from build123d import *

# Parameters (mm, degrees)
CROQUIS1_R              = 1.5875
SALIENTE_EXTRUIR1_DEPTH = 3.175
CORTAR_EXTRUIR1_DEPTH   = 3.175
CORTAR_EXTRUIR3_DEPTH   = 10
CORTAR_EXTRUIR4_DEPTH   = 10
BOSS_EXTRU_1_DEPTH      = 8.18
CONG_1_R                = 2
CONG_2_R                = 3


with BuildPart() as part:
    # Croquis1 → Saliente-Extruir1 (new body)
    with BuildSketch(Plane(origin=(0, 0, 0), x_dir=(1, 0, 0), z_dir=(0, 1, 0))):
        with BuildLine():
            Line((-12.5, 0), (-12.5, -40))
            Line((-12.5, -40), (-2.975, -40))
            Line((-2.975, -40), (-2.975, -20))
            ThreePointArc((-2.975, -20), (-0.046067812, -12.928932188), (7.025, -10))
            Line((7.025, -10), (12.5, -10))
            Line((12.5, -10), (12.5, 40))
            Line((12.5, 40), (2.5, 40))
            Line((2.5, 40), (-12.5, 0))
        make_face()
        with Locations(Location((-7.7375, -5, 0), (0, 0, 270))):
            Circle(CROQUIS1_R, mode=Mode.SUBTRACT)
        with Locations(Location((-7.7375, -35, 0), (0, 0, 270))):
            Circle(CROQUIS1_R, mode=Mode.SUBTRACT)
    extrude(amount=SALIENTE_EXTRUIR1_DEPTH)

    # Croquis2 → Cortar-Extruir1 (cut)
    with BuildSketch(Plane(origin=(0, 3.175, 0), x_dir=(1, 0, 0), z_dir=(0, 1, 0))):
        Polygon((12.5, -10), (6.1, 40), (12.5, 40), align=None)
    extrude(amount=-CORTAR_EXTRUIR1_DEPTH, mode=Mode.SUBTRACT)

    # Croquis3 → Cortar-Extruir3 (cut)
    with BuildSketch(Plane(origin=(0, 3.175, 0), x_dir=(1, 0, 0), z_dir=(0, 1, 0))):
        with BuildLine():
            ThreePointArc((-5.975, -30.575635639), (-7.7375, -30.2375), (-9.5, -30.575635639))
            Line((-9.5, -30.575635639), (-9.5, -9.427055314))
            ThreePointArc((-9.5, -9.427055314), (-7.7375, -9.765), (-5.975, -9.427055314))
            Line((-5.975, -9.427055314), (-5.975, -14.803847577))
            Line((-5.975, -14.803847577), (-5.975, -30.575635639))
        make_face()
        with BuildLine():
            ThreePointArc((-12.5, -35), (-7.7375, -39.7625), (-2.975, -35))
            Line((-2.975, -35), (-2.975, -40))
            Line((-2.975, -40), (-12.5, -40))
            Line((-12.5, -40), (-12.5, -35))
        make_face()
    extrude(amount=-CORTAR_EXTRUIR3_DEPTH, mode=Mode.SUBTRACT)

    # Croquis4 → Cortar-Extruir4 (cut)
    with BuildSketch(Plane(origin=(0, 3.175, 0), x_dir=(1, 0, 0), z_dir=(0, 1, 0))):
        Polygon((7.025, -10), (11.878723404, -5.146276596), (12.5, -10), align=None)
    extrude(amount=-CORTAR_EXTRUIR4_DEPTH, mode=Mode.SUBTRACT)

    # Esquisse1 → Boss.-Extru.1 (add)
    with BuildSketch(Plane(origin=(0, 3.175, 0), x_dir=(1, 0, 0), z_dir=(0, 1, 0))):
        Polygon((11.878723404, -5.146276596), (6.1, 40), (2.5, 40), (8.687234043, -8.337765957), align=None)
    extrude(amount=-BOSS_EXTRU_1_DEPTH)

    # Congé1
    cong_1_edges = [part.edges().sort_by_distance(p)[0] for p in [
        (5.593617021, -5.005, -15.831117021),
    ]]
    fillet(cong_1_edges, radius=CONG_1_R)

    # Congé2
    cong_2_edges = [part.edges().sort_by_distance(p)[0] for p in [
        (5.593617021, 0, -15.831117021),
    ]]
    fillet(cong_2_edges, radius=CONG_2_R)


solid = part.part
Geometry: final body of the model. Coordinates: model frame, mm. A direction names the side the tool comes from. Coordinates: 2 decimals unless noted, no trailing zeros. Write each loop counter-clockwise with the first axis right and the second up, starting at its lowest first coordinate (ties: lowest second). Pieces come first, ordered by that corner, then holes. Notation, with made-up numbers: (38.5, 28) - (94.5, 28) arc R13 cw to (94.5, 34) - close; hole circle Ø2 at (86.25, -15). An arc over 180 degrees is marked (long way). Return JSON: item names as keys, results as strings.
Item 1: Section query C-C (x = -1.5). Output: boundary loops of the cut face in (y, z) (3 decimals), and give its area (3 significant figures).
Completed:
{"outline": "(0, -29.333) - (3.175, -29.333) - (3.175, 14.773) - (0, 14.773) - close", "area": "140 mm2"}
Item 2: Reachability of faces 1 (the face through (-2.975, 2, 28)), 2 (the face through (8, -5.005, -19)), 3 (the face through (-5.975, 2, 20)) from +Z, -Z, +X, -X, +Y, -Y: full face, straight path, thin tool, end or side. Return the list, or none.
Completed:
{"face 1": "+Z, +X, +Y, -Y", "face 2": "+Z, -Z, +X, -X, -Y", "face 3": "+Y, -Y"}
Item 3: Section query D-D (y = -1.75). Output: boundary loops of the cut face in (x, z), and give its area (3 significant figures).
Completed:
{"outline": "(2.29, -39.45) - (2.5, -40) - (6.1, -40) - (11.88, 5.15) - (8.44, 8.58) - close", "area": "182 mm2"}
Item 4: Pin query (flat end, axial travel): pin 1 Ø1.6 at (y, z) = (1, 24.5) entering from +X (3 decimals); pin 2 Ø3 at (x, z) = (0, -12) entering from -Y; pin 3 Ø3 at (x, z) = (-7.74, 5) entering from +Y; pin 4 Ø1 at (y, z) = (2, 18.5) entering from +X. Return the tip coordinate at first contact, or that it passes through.
Completed:
{"pin 1": "stops at x = -2.975", "pin 2": "stops at y = 0", "pin 3": "passes through", "pin 4": "stops at x = -2.77"}
Item 5: Section query B-B (y = 1.25). Output: boundary loops of the cut face in (x, z) (1 decimal), and give its area (3 significant figures).
Completed:
{"outline": "(-12.5, 0) - (2.5, -40) - (6.1, -40) - (11.9, 5.1) - (7, 10) arc R10 cw to (-3, 20) - (-3, 35) arc R4.8 ccw to (-12.5, 35) - close; hole (-9.5, 9.4) arc R4.8 cw to (-6, 9.4) - (-6, 30.6) arc R4.8 cw to (-9.5, 30.6) - close; hole circle Ø3.2 at (-7.7, 5); hole circle Ø3.2 at (-7.7, 35)", "area": "983 mm2"}
Item 6: Section query A-A (z = 25.5). Output: boundary loops of the cut face in (x, y) (3 decimals).
Completed:
{"outline": "(-12.5, 0) - (-9.5, 0) - (-9.5, 3.175) - (-12.5, 3.175) - close; (-5.975, 0) - (-2.975, 0) - (-2.975, 3.175) - (-5.975, 3.175) - close"}
Item 7: Line query: L1, parallel to X at y = 1.85, z = 35 (3 decimals); L2, parallel to Y at x = 5.5, z = 8.5 (3 decimals); L3, parallel to X at y = 2.5, z = 27 (3 decimals). Output: solid intervals per line, ascending.
Completed:
{"L1": "x = -12.5 to -9.325, -6.15 to -2.975", "L2": "y = 0 to 3.175", "L3": "x = -12.5 to -9.5, -5.975 to -2.975"}
Item 8: Pull-direction query (Z, two-part tool) for faces 4 (the face through (-7.712, 1.61, 30.238)), 5 (the face through (6.23, -4.43, -15.57)), 6 (the face through (0, 3.175, -1)), 7 (the face through (-5, 1, -20)); classes: +Z half, -Z half, draft (parallel to the pull), parting line (faces both ways), or undercut.
Completed:
{"face 4": "undercut", "face 5": "+Z half", "face 6": "draft", "face 7": "-Z half"}
